Source: CAD feature listing. Evaluate the final solid. Frame: model axes, mm. Round coordinates to 2 decimals unless told otherwise and drop trailing zeros. Loops run counter-clockwise (first coordinate to the right, second up) from the corner with the lowest first, then second, coordinate; pieces in that order, holes last. Notation, with made-up numbers: M -13.75,-24 L 41.25,-24 A20 cw 41.25,0 Z; hole C 22.25,1.25 d8. An arc over 180 degrees is marked long. Write each question's results on one line, items separated by ' | '. Start each with the question number.
1. Section A-A on z = 35.5. Output: boundary loops of the cut face in (x, y), and give its area (3 significant figures).
2. Contact query for flat-ended pins moving along their axis: pin 1 Ø3 at (y, z) = (-6.5, 8.5) entering from -X; pin 2 Ø10 at (y, z) = (-12, 20.5) entering from -X; pin 3 Ø6 at (y, z) = (-10, 36.5) entering from -X. Output: stop coordinate, or through.
3. Ray query, line 1 (X direction, y = 18.5, z = 37.5); line 2 (X direction, y = 12, z = 9); line 3 (Y direction, x = -79, z = 44). Return the intervals inside material, ascending.
Autodesk Inventor part; units mm, degrees
ref_plane "YZ Plane" through (0, 0, 0) normal (1, 0, 0) x (0, 1, 0)
ref_plane "XZ Plane" through (0, 0, 0) normal (0, 1, 0) x (-1, 0, 0)
ref_plane "XY Plane" through (0, 0, 0) normal (0, 0, 1) x (1, 0, 0)
sketch "Boceto1" plane through (0, 0, 0) normal (0, 0, 1) x (1, 0, 0)
  line L0 (100, -20) -> (-100, -20)
  line L1 (-60, 20) -> (100, 20)
  line L2 (100, 20) -> (100, -20)
  line L3 (100, -20) -> (-66.6667, 13.3333) construction
  line L4 (-100, -20) -> (100, 20) construction
  line L5 (-100, -20) -> (-60, 20)
  line L6 (-100, -20) -> (-43.4315, -20) construction
  point P0 (0, 0)
  dimension "d2" = 45
extrude "Extrusión1" add sketch "Boceto1" along normal blind 80
fillet "Empalme1" radius 2 11 edges at (20, 20, 0) (20, 20, 80) (0, -20, 0) (0, -20, 80) (-80, 0, 80) (-60, 20, 40) (-80, 0, 0) (100, 20, 40) (100, 0, 80) (100, 0, 0) (100, -20, 40)
properties part number "union_ruedas" material "Hierro, fundido"
Taken from the geometry:
1) outline: M -100,-20 L 98,-20 A2 ccw 100,-18 L 100,18 A2 ccw 98,20 L -59.17,20 A2 ccw -60.59,19.41 Z | area: 7,200 mm^2
2) pin 1: x = -88 | pin 2: x = -97 | pin 3: x = -93
3) line 1: -61.5 to 99.94 | line 2: -68 to 100 | line 3: -20 to 1
